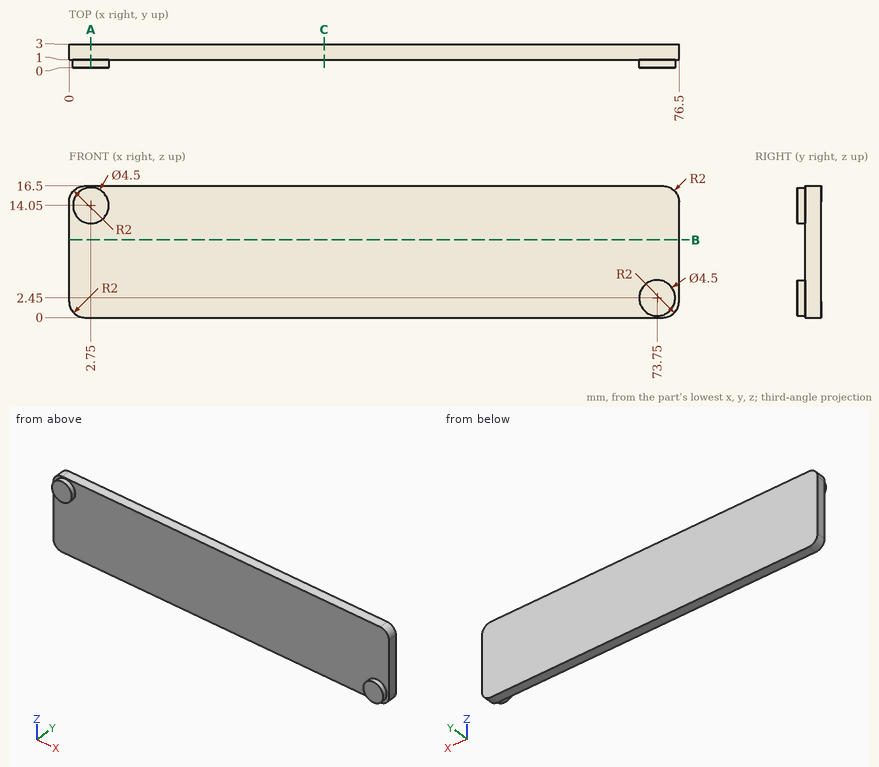
The figure shows three views and two pictorial views of one solid part (mm, origin at its lowest corner). Answer the questions. Round coordinates to 2 decimals unless told otherwise and drop trailing zeros. Loops run counter-clockwise (first coordinate to the right, second up) from the corner with the lowest first, then second, coordinate; pieces in that order, holes last. Notation, with made-up numbers: M 83,1 L 118,1 A23 cw 118,12 Z; hole C -22,64 d2. An arc over 180 degrees is marked long. Use CSV: the item, a comma, the result in double quotes.
Q1. Section B-B, the plane z = 9.75 is taken. Determine the outline of the cut face in (x, y).
Determined:
outline,"M 0,1 L 76.5,1 L 76.5,3 L 0,3 Z"
Q2. Section C-C, the plane x = 32 is taken. Determine the outline of the cut face in (y, z), then the cut area to 3 significant figures.
Determined:
outline,"M 1,0 L 3,0 L 3,16.5 L 1,16.5 Z"
area,"33.0 mm2"
Q3. Consider L1, parallel to Y at x = 12.5, z = 1.5; L2, parallel to X at y = 0.25, z = 3.75; L3, parallel to X at y = 0.4, z = 14.75. Determine where each line is inside the solid, lowest interval first.
Determined:
L1,"1 to 3"
L2,"71.91 to 75.59"
L3,"0.61 to 4.89"
Q4. Section A-A, the plane x = 2.75 is taken. Determine the outline of the cut face in (y, z), then the cut area to 3 significant figures.
Determined:
outline,"M 0,11.8 L 1,11.8 L 1,0 L 3,0 L 3,16.5 L 1,16.5 L 1,16.3 L 0,16.3 Z"
area,"37.5 mm2"
Q5. This flat-tipped pin is pushed along its axis until it touches: pin 1 (2 mm diameter, centred on x = 53.5, z = 10.5, fed in from -Y). Where does it stop, or does it pass through?
Determined:
pin 1,"y = 1"
